from build123d import *

# Parameters (mm, degrees)
TABAN_FLAN_1_DEPTH    = 10
IZIM2_R               = 25
IZIM2_R_2             = 4.25
IZIM2_R_3             = 5.5
IZIM2_R_4             = 3.25
KES_EKSTR_ZYON1_DEPTH = 10
RADYUS3_R             = 30
RADYUS4_R             = 10
RADYUS5_R             = 50
IZIM3_R               = 3.25
KES_EKSTR_ZYON2_DEPTH = 10
RADYUS7_R             = 10
RADYUS8_R             = 30


# Sheet-metal steps are written as plain solids
with BuildPart() as part:
    # Çizim1 → Taban-Flanş1 (new body)
    with BuildSketch(Plane.XY):
        Polygon((0, 120), (-470, 120), (-470, -55), (-410, -55), (-380, -40), (-300, -40), (-250, -30), (-185, -30), (-185, -90), (-150, -90), (-150, -30), (0, -30), (0, 0), align=None)
    extrude(amount=-TABAN_FLAN_1_DEPTH)

    # Çizim2 → Kes-Ekstrüzyon1 (cut)
    with BuildSketch(Plane.XY):
        with Locations((-360, 45)):
            Circle(IZIM2_R)
        with Locations((-401.5, 86.5)):
            Circle(IZIM2_R_2)
        with Locations((-318.5, 86.5)):
            Circle(IZIM2_R_2)
        with Locations((-401.5, 3.5)):
            Circle(IZIM2_R_2)
        with Locations((-318.5, 3.5)):
            Circle(IZIM2_R_2)
        with Locations((-110, 55)):
            Circle(IZIM2_R_3)
        with Locations((-210, 55)):
            Circle(IZIM2_R_3)
        with Locations((-210, 15)):
            Circle(IZIM2_R_3)
        with Locations((-110, 15)):
            Circle(IZIM2_R_3)
        with Locations((-167.5, -75)):
            Circle(IZIM2_R_3)
        with Locations((-455, 10)):
            Circle(IZIM2_R_4)
        with Locations((-455, -40)):
            Circle(IZIM2_R_4)
    extrude(amount=-KES_EKSTR_ZYON1_DEPTH, mode=Mode.SUBTRACT)

    # Radyus3
    radyus3_edges = [part.edges().sort_by_distance(p)[0] for p in [
        (0, 120, -5),
    ]]
    fillet(radyus3_edges, radius=RADYUS3_R)

    # Radyus4
    radyus4_edges = [part.edges().sort_by_distance(p)[0] for p in [
        (0, -30, -5),
        (-150, -30, -5),
        (-150, -90, -5),
        (-185, -90, -5),
        (-185, -30, -5),
    ]]
    fillet(radyus4_edges, radius=RADYUS4_R)

    # Radyus5
    radyus5_edges = [part.edges().sort_by_distance(p)[0] for p in [
        (-250, -30, -5),
        (-300, -40, -5),
        (-380, -40, -5),
        (-410, -55, -5),
    ]]
    fillet(radyus5_edges, radius=RADYUS5_R)

    # Çizim3 → Kes-Ekstrüzyon2 (cut)
    with BuildSketch(Plane(origin=(0, 0, -10), x_dir=(-1, 0, 0), z_dir=(0, 0, -1))):
        with Locations((277, 92.5)):
            Circle(IZIM3_R)
        with Locations((277, 12.5)):
            Circle(IZIM3_R)
        with Locations((445, 37.5)):
            Circle(IZIM3_R)
        with Locations((445, 92.5)):
            Circle(IZIM3_R)
        with Locations((140, 92)):
            Circle(IZIM3_R)
        with Locations((35, 92)):
            Circle(IZIM3_R)
        with Locations((35, 32)):
            Circle(IZIM3_R)
        with Locations((140, 32)):
            Circle(IZIM3_R)
    extrude(amount=-KES_EKSTR_ZYON2_DEPTH, mode=Mode.SUBTRACT)

    # Radyus7
    radyus7_edges = [part.edges().sort_by_distance(p)[0] for p in [
        (-470, -55, -5),
    ]]
    fillet(radyus7_edges, radius=RADYUS7_R)

    # Radyus8
    radyus8_edges = [part.edges().sort_by_distance(p)[0] for p in [
        (-470, 120, -5),
    ]]
    fillet(radyus8_edges, radius=RADYUS8_R)


solid = part.part
Geometry: final body of the model. Coordinates: model frame, mm. A direction names the side the tool comes from. Give positions to 0.01 mm unless a question says otherwise; leave off trailing zeros. Loops run counter-clockwise (first coordinate to the right, second up) from the corner with the lowest first, then second, coordinate; pieces in that order, holes last. Notation, with made-up numbers: (76, 55.5) - (117, 55.5) arc R22 ccw to (117, 67.5) - close; hole circle Ø10 at (-16, 17.5). An arc over 180 degrees is marked (long way). Answer as CSV lines item,"result". Start each with the question number.
1. Section B-B, the plane y = -75. Return loops of the section in (x, z).
2. Draft query along X for faces 1 (the face through (-181.99, -87.15, -5.07)), 2 (the face through (-173, -75, -5)), 3 (the face through (-2.85, -26.99, -5.07)). Return one class per face: released by +X, released by -X, zero draft, split by the parting line, or undercut.
3. Reachability of faces 4 (the face through (-405.746, 3.687, -4.93)), 5 (the face through (-76, -30, -5)), 6 (the face through (-337, -40, -5)) from +Z, -Z, +X, -X, +Y, -Y: full face, straight path, thin tool, end or side. Return the list, or none.
4. Section A-A, the plane x = -360. Return loops of the section in (y, z).
5. Pin query (flat end, axial travel): P1, Ø5, axis at x = -51.5, z = -4, coming from the -Y side; P2, Ø4, axis at x = -343, z = -3, coming from the -Y side; P3, Ø2, axis at y = 94, z = -7.5, coming from the +X side. Return the tip coordinate at first contact, or that it passes through.
6. Ray query, L1, parallel to Y at x = -318.5, z = -2.25; L2, parallel to Y at x = -110, z = -4.25; L3, parallel to X at y = 56.5, z = -0.25. Return the intervals inside material, ascending.
7. Section D-D, the plane z = -1.5. Give the number of separate pieces and of enclosed holes in the cut face, plus the area to 3 significant figures.
8. Section C-C, the plane x = -210. Return loops of the section in (y, z), plus the area to 3 significant figures.
Answers:
1,outline,"(-185, -10) - (-173, -10) - (-173, 0) - (-185, 0) - close; (-162, -10) - (-150, -10) - (-150, 0) - (-162, 0) - close"
2,face 1,"released by -X"
2,face 2,"undercut"
2,face 3,"released by +X"
3,face 4,"+Z, -Z"
3,face 5,"+Z, -Z, +X, -Y"
3,face 6,"+Z, -Z, -Y"
4,outline,"(-40, -10) - (20, -10) - (20, 0) - (-40, 0) - close; (70, -10) - (120, -10) - (120, 0) - (70, 0) - close"
5,P1,"stops at y = -30"
5,P2,"stops at y = -40"
5,P3,"stops at x = -0.15"
6,L1,"y = -40 to -0.75, 7.75 to 82.25, 90.75 to 120"
6,L2,"y = -30 to 9.5, 20.5 to 49.5, 60.5 to 120"
6,L3,"x = -470 to -382.2, -337.8 to -215.29, -204.71 to -115.29, -104.71 to 0"
7,separate pieces,"1"
7,enclosed holes,"20"
7,area,"72,200 mm2"
8,outline,"(-30, -10) - (9.5, -10) - (9.5, 0) - (-30, 0) - close; (20.5, -10) - (49.5, -10) - (49.5, 0) - (20.5, 0) - close; (60.5, -10) - (120, -10) - (120, 0) - (60.5, 0) - close"
8,area,"1,280 mm2"
